Could you check a few things on this model? Use its own coordinates, in mm. Face numbers are marked on the shaded views. Give positions to 0.01 mm unless a question says otherwise; leave off trailing zeros. Loops run counter-clockwise (first coordinate to the right, second up) from the corner with the lowest first, then second, coordinate; pieces in that order, holes last. Notation, with made-up numbers: (37.25, 15.25) - (67.25, 15.25) arc R11 ccw to (67.25, 29.25) - close; hole circle Ø10 at (25.5, 2). An arc over 180 degrees is marked (long way). Write each question's results on one line, items separated by ' | '. Start each with the question number.
1) I want a section at A-A, the plane y = 1.25. Write out the boundary of the cut face in (x, z).
2) I want a section at C-C, the plane y = -9.5. Write out the boundary of the cut face in (x, z), and give its area (3 significant figures).
3) I want a section at D-D, the plane z = 17.5. Write out the boundary of the cut face in (x, y).
4) I want a section at B-B, the plane x = 15.5. Write out the boundary of the cut face in (y, z), and give its area (3 significant figures).
5) I'm going to push flat-ended pins straight in: pin 1 (2 mm diameter, centred on y = 2, z = -3, fed in from +X); pin 2 (3 mm diameter, centred on y = -8.5, z = -16.5, fed in from +X); pin 3 (4.5 mm diameter, centred on x = 15.32, z = 16, fed in from -Y); pin 4 (5.5 mm diameter, centred on x = 16.5, z = 15.5, fed in from -Y). Where does each tip first touch, or does it pass through?
6) If we mould it in two halves opening along X, with no side actions, what happens to the marked faces 1, 2 and 3? For each: +X half, -X half, draft (parallel to the pull), parting line (faces both ways), or undercut.
7) If I drill on probe 1 along Z at (x, y) = (-16, -11.5); probe 2 along Z at (x, y) = (2.5, 8.75); probe 3 along X at (y, z) = (-9.5, 8.5), over which ranges is the centre line in solid material (lowest first)? Write a range as [from, to].
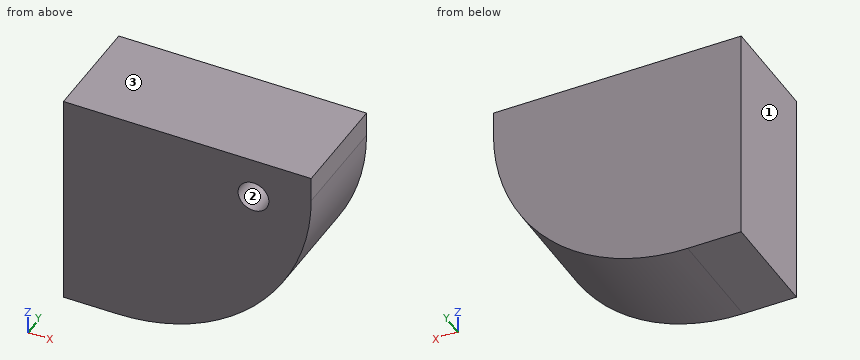
from build123d import *

# Parameters (mm, degrees)
F0_W     = 57.3965907097
F0_H     = 50.7467389107
F1_DEPTH = 12.5
F3_D     = 7.1374
F3_DEPTH = 12.501
F4_R     = 45


with BuildPart() as f1:
    # F0 (on Front) → F1 (new body, symmetric)
    with BuildSketch(Plane.XZ):
        Rectangle(F0_W, F0_H)
    extrude(amount=F1_DEPTH, both=True)

    # F3 (through all, one way)
    with BuildSketch(Plane(origin=(0, 0, 0), x_dir=(1, 0, 0), z_dir=(0, 1, 0))):
        with Locations((15.3181608766, -16.0046312958)):
            Circle(F3_D / 2)
    extrude(amount=-F3_DEPTH, mode=Mode.SUBTRACT)

    # F4
    f4_edges = [f1.edges().sort_by_distance(p)[0] for p in [
        (28.698295, 0, -25.373369),
    ]]
    fillet(f4_edges, radius=F4_R)


solid = f1.part
Answers:
1) outline: (-28.7, -25.37) - (-16.3, -25.37) arc R45 ccw to (28.7, 19.63) - (28.7, 25.37) - (-28.7, 25.37) - close
2) outline: (-28.7, -25.37) - (-16.3, -25.37) arc R45 ccw to (28.7, 19.63) - (28.7, 25.37) - (-28.7, 25.37) - close; hole circle Ø7.14 at (15.32, 16) | area: 2,440 mm2
3) outline: (-28.7, -12.5) - (12.08, -12.5) - (12.08, 0) - (18.56, 0) - (18.56, -12.5) - (28.65, -12.5) - (28.65, 12.5) - (-28.7, 12.5) - close
4) outline: (-12.5, -12.21) - (12.5, -12.21) - (12.5, 25.37) - (-12.5, 25.37) - (-12.5, 19.57) - (0, 19.57) - (0, 12.44) - (-12.5, 12.44) - close | area: 851 mm2
5) pin 1: stops at x = 23.16 | pin 2: stops at x = 12.44 | pin 3: stops at y = 0 | pin 4: stops at y = -12.5
6) face 1: -X half | face 2: undercut | face 3: draft
7) probe 1: z = [-25.37, 25.37] | probe 2: z = [-21.26, 25.37] | probe 3: x = [-28.7, 27.3]
